Build history of the part. All positions in model axes, mm. Face numbers are marked on the shaded views. A direction names the side the tool comes from. Give positions to 0.01 mm unless a question says otherwise; leave off trailing zeros. Loops run counter-clockwise (first coordinate to the right, second up) from the corner with the lowest first, then second, coordinate; pieces in that order, holes last. Notation, with made-up numbers: (85, 20) -> (99, 20) arc R36 cw to (99, 55) -> close; hole circle Ø5 at (59.25, 65). An arc over 180 degrees is marked (long way). Answer as a JSON object with one key per item and string values. Group by question number.
Q1. Band-saw the part on C-C, the plane y = 6. Write the cut outline in (x, z).
Q2. Band-saw the part on A-A, the plane x = 0. Write the cut outline in (y, z).
Q3. Wall check: probe 1 along X at (y, z) = (0.05, 0); probe 2 along Y at (x, z) = (0.6, -0.85); probe 3 along Y at (x, z) = (0.8, 1.3). Give the ranges that are in metal, low to high. Write a range as from..to.
Q4. Two-plate mould, pull along X, no slides. Class the marked faces 1, 2, 3 and 4: pulls with the +X half, pulls with the -X half, needs draft (parallel to the pull), parting line crosses it, or undercut.
Q5. Tool access for the marked faces 5 and 6: list every direction of +Z, -Z, +X, -X, +Y, -Y with a clear straight run to the whole face (end or side of a thin tool).
Q6. Band-saw the part on B-B, the plane z = 0. Write the cut outline in (x, y), plus the area to 4 significant figures.
from build123d import *

# Parameters (mm, degrees)
SKETCH_1_W          = 3
SKETCH_1_H          = 3
EXTRUDE_1_DEPTH     = 4.4
SKETCH_2_R          = 1.4
EXTRUDE_2_DEPTH     = 2
SKETCH_3_R          = 1.1
CUT_EXTRUDE_1_DEPTH = 0.2
CHAMFER_1_SIZE      = 0.1
SKETCH_4_W          = 3.5
SKETCH_4_H          = 3.5
SKETCH_4_W_2        = 3
SKETCH_4_H_2        = 3
EXTRUDE_3_DEPTH     = 4.4


with BuildPart() as part:
    # 草图1 → 凸台-拉伸1 (new body)
    with BuildSketch(Plane(origin=(0, 0, 0), x_dir=(1, 0, 0), z_dir=(0, 1, 0))):
        Rectangle(SKETCH_1_W, SKETCH_1_H)
    extrude(amount=EXTRUDE_1_DEPTH)

    # 草图2 → 凸台-拉伸2 (add)
    with BuildSketch(Plane(origin=(0, 4.4, 0), x_dir=(1, 0, 0), z_dir=(0, 1, 0))):
        with Locations(Location((0, 0, 0), (0, 0, 90))):
            Circle(SKETCH_2_R)
    extrude(amount=EXTRUDE_2_DEPTH)

    # 草图3 → 切除-拉伸1 (cut)
    with BuildSketch(Plane.XZ):
        with Locations(Location((0, 0, 0), (0, 0, 270))):
            Circle(SKETCH_3_R)
    extrude(amount=-CUT_EXTRUDE_1_DEPTH, mode=Mode.SUBTRACT)

    # 倒角1
    chamfer_1_edges = [part.edges().sort_by_distance(p)[0] for p in [
        (0, 6.4, 1.4),
    ]]
    chamfer(chamfer_1_edges, length=CHAMFER_1_SIZE)

    # 草图4 → 凸台-拉伸3 (add)
    with BuildSketch(Plane.XZ):
        Rectangle(SKETCH_4_W, SKETCH_4_H)
        Rectangle(SKETCH_4_W_2, SKETCH_4_H_2, mode=Mode.SUBTRACT)
    extrude(amount=-EXTRUDE_3_DEPTH)


solid = part.part
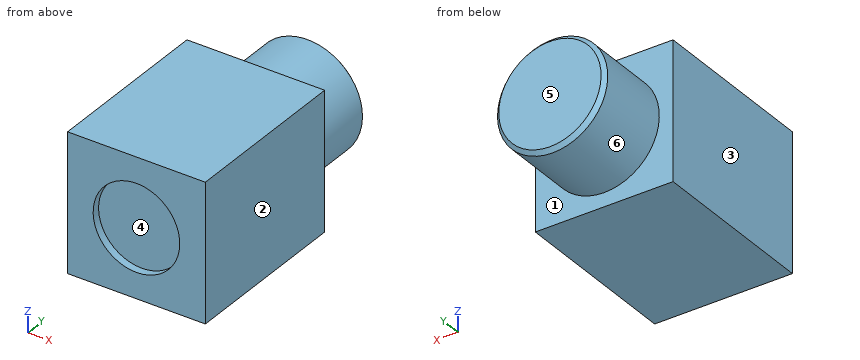
Worked answers:
{
 "1": {"outline": "circle Ø2.8 at (0, 0)"},
 "2": {"outline": "(0, -1.75) -> (4.4, -1.75) -> (4.4, -1.4) -> (6.3, -1.4) -> (6.4, -1.3) -> (6.4, 1.3) -> (6.3, 1.4) -> (4.4, 1.4) -> (4.4, 1.75) -> (0, 1.75) -> (0, 1.1) -> (0.2, 1.1) -> (0.2, -1.1) -> (0, -1.1) -> close"},
 "3": {"probe 1": "-1.75..-1.1, 1.1..1.75", "probe 2": "0.2..6.4", "probe 3": "0..4.4"},
 "4": {"face 1": "needs draft", "face 2": "pulls with the +X half", "face 3": "pulls with the -X half", "face 4": "undercut"},
 "5": {"face 5": "+Z, -Z, +X, -X, +Y", "face 6": "+Y"},
 "6": {"outline": "(-1.75, 0) -> (-1.1, 0) -> (-1.1, 0.2) -> (1.1, 0.2) -> (1.1, 0) -> (1.75, 0) -> (1.75, 4.4) -> (1.4, 4.4) -> (1.4, 6.3) -> (1.3, 6.4) -> (-1.3, 6.4) -> (-1.4, 6.3) -> (-1.4, 4.4) -> (-1.75, 4.4) -> close", "area": "20.55 mm2"}
}
